from build123d import *

# Parameters (mm, degrees)
SKETCH1_W           = 23
SKETCH1_H           = 23
BOSS_EXTRUDE1_DEPTH = 1.2
FILLET1_R           = 1
SKETCH2_W           = 5
SKETCH2_H           = 4
BOSS_EXTRUDE2_DEPTH = 1.75
FILLET2_R           = 0.3
SKETCH4_R           = 1.65
CUT_EXTRUDE1_DEPTH  = 1.75


with BuildPart() as part:
    # Sketch1 → Boss-Extrude1 (new body)
    with BuildSketch(Plane(origin=(0, 0, 0), x_dir=(1, 0, 0), z_dir=(0, 1, 0))):
        Rectangle(SKETCH1_W, SKETCH1_H)
    extrude(amount=BOSS_EXTRUDE1_DEPTH)

    # Fillet1
    fillet1_edges = [part.edges().sort_by_distance(p)[0] for p in [
        (11.5, 0.6, 11.5),
        (-11.5, 0.6, 11.5),
        (-11.5, 0.6, -11.5),
        (11.5, 0.6, -11.5),
    ]]
    fillet(fillet1_edges, radius=FILLET1_R)

    # Sketch2 → Boss-Extrude2 (add)
    with BuildSketch(Plane(origin=(0, 1.2, 0), x_dir=(1, 0, 0), z_dir=(0, 1, 0))):
        Rectangle(SKETCH2_W, SKETCH2_H)
    extrude(amount=BOSS_EXTRUDE2_DEPTH)

    # Fillet2
    fillet2_edges = [part.edges().sort_by_distance(p)[0] for p in [
        (2.5, 2.075, 2),
        (2.5, 2.075, -2),
        (-2.5, 2.075, -2),
        (-2.5, 2.075, 2),
        (2.5, 2.95, 0),
        (0, 2.95, -2),
        (-2.5, 2.95, 0),
        (0, 2.95, 2),
    ]]
    fillet(fillet2_edges, radius=FILLET2_R)

    # Sketch4 → Cut-Extrude1 (cut)
    with BuildSketch(Plane(origin=(0, 1.2, 0), x_dir=(1, 0, 0), z_dir=(0, 1, 0))):
        with Locations(Location((-8, 8, 0), (0, 0, 270))):
            Circle(SKETCH4_R)
        with Locations(Location((8, 8, 0), (0, 0, 270))):
            Circle(SKETCH4_R)
        with Locations(Location((8, -8, 0), (0, 0, 270))):
            Circle(SKETCH4_R)
        with Locations(Location((-8, -8, 0), (0, 0, 270))):
            Circle(SKETCH4_R)
    extrude(amount=-CUT_EXTRUDE1_DEPTH, mode=Mode.SUBTRACT)


solid = part.part
For this review, take the finished solid that the model builds, in its own axes (mm). A direction names the side the tool comes from. Give positions to 0.01 mm unless a question says otherwise; leave off trailing zeros. Order: outer loops, then holes, each group sorted by start corner. A loop starts at its lowest first (then second) coordinate and runs counter-clockwise, first axis right, second up. Notation, with made-up numbers: (-18.5, 56) - (14.5, 56) arc R21 cw to (14.5, 83) - close; hole circle Ø9 at (16.5, 19.25). An arc over 180 degrees is marked (long way). Answer as a JSON object with one key per item and string values. Group by question number.
Item 1: Draft analysis for pull direction Z (two halves, no side actions). For faces 4 (the cylindrical face through (11.199, 0.608, 11.215)), 5 (the flat face through (2.5, 2, 0)), 6 (the cylindrical face through (-7.93, 0.61, -9.65)), state which applies: pulls with the +Z half, pulls with the -Z half, needs draft (parallel to the pull), parting line crosses it, or undercut.
Item 2: Take a section at A-A on z = -8. Give the boundary of the cut face in (x, y).
Item 3: Clearance check with flat-ended pins moving along their axes: pin 1 Ø5.5 at (x, z) = (-8, -8) entering from +Y; pin 2 Ø1.5 at (y, z) = (2, -8.5) entering from -X; pin 3 Ø0.7 at (y, z) = (2, 0.5) entering from -X; pin 4 Ø1.2 at (x, y) = (1, 2) entering from +Z. State where each tip first meets the part, or that it passes through.
Item 4: Take a section at C-C on z = -0.75. Give the boundary of the cut face in (x, y), and give its area (3 significant figures).
Item 5: Take a section at D-D on x = 1.75. Give the boundary of the cut face in (y, z).
Item 6: Take a section at B-B on x = -8. Give the boundary of the cut face in (y, z).
Item 7: Machinability: for faces 1 (the flat face through (0, 2, 2)), 2 (the flat face through (-2.5, 2, 0)), 3 (the flat face through (0, 2, -2)), which of the approach directions +Z, -Z, +X, -X, +Y, -Y give a long, thin tool a straight path to every point of the face, cutting with its end or side? Answer none if there is none.
Item 8: Wall thickness on line 1 along X through (y, z) = (0.75, 8); line 2 along X through (y, z) = (0.4, 9); line 3 along Z through (x, y) = (6.75, 0.5): over which ranges is each line inside the solid? List them lowest first.
Reported:
{
 "1": {"face 4": "pulls with the +Z half", "face 5": "needs draft", "face 6": "undercut"},
 "2": {"outline": "(-11.5, 0) - (-9.65, 0) - (-9.65, 1.2) - (-11.5, 1.2) - close; (-6.35, 0) - (6.35, 0) - (6.35, 1.2) - (-6.35, 1.2) - close; (9.65, 0) - (11.5, 0) - (11.5, 1.2) - (9.65, 1.2) - close"},
 "3": {"pin 1": "y = 1.2", "pin 2": "through", "pin 3": "x = -2.5", "pin 4": "z = 2"},
 "4": {"outline": "(-11.5, 0) - (11.5, 0) - (11.5, 1.2) - (2.5, 1.2) - (2.5, 2.65) arc R0.3 ccw to (2.2, 2.95) - (-2.2, 2.95) arc R0.3 ccw to (-2.5, 2.65) - (-2.5, 1.2) - (-11.5, 1.2) - close", "area": "36.3 mm^2"},
 "5": {"outline": "(0, -11.5) - (1.2, -11.5) - (1.2, -2) - (2.65, -2) arc R0.3 ccw to (2.95, -1.7) - (2.95, 1.7) arc R0.3 ccw to (2.65, 2) - (1.2, 2) - (1.2, 11.5) - (0, 11.5) - close"},
 "6": {"outline": "(0, -11.5) - (1.2, -11.5) - (1.2, -9.65) - (0, -9.65) - close; (0, -6.35) - (1.2, -6.35) - (1.2, 6.35) - (0, 6.35) - close; (0, 9.65) - (1.2, 9.65) - (1.2, 11.5) - (0, 11.5) - close"},
 "7": {"face 1": "+Z, +X, -X, +Y", "face 2": "+Z, -Z, -X, +Y", "face 3": "-Z, +X, -X, +Y"},
 "8": {"line 1": "-11.5 to -9.65, -6.35 to 6.35, 9.65 to 11.5", "line 2": "-11.5 to -9.31, -6.69 to 6.69, 9.31 to 11.5", "line 3": "-11.5 to -9.08, -6.92 to 6.92, 9.08 to 11.5"}
}
